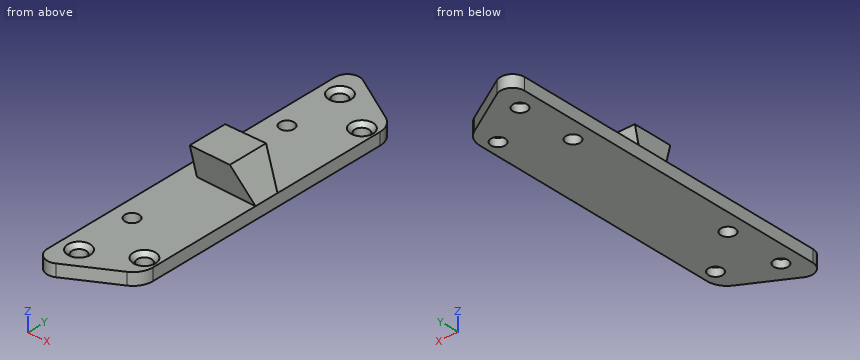
Autodesk Inventor part; units mm, degrees
ref_plane "Plano de trabajo1" through (130.1908, -31.0595, 0) normal (1, 0, 0) x (0, 0, -1)
ref_plane "YZ Plane" through (0, 0, 0) normal (1, 0, 0) x (0, 1, 0)
ref_plane "XZ Plane" through (0, 0, 0) normal (0, 1, 0) x (-1, 0, 0)
sketch "Boceto1" plane through (0, 0, 0) normal (0, 0, 1) x (1, 0, 0)
  line L0 (134.9, 24.045) -> (134.9, 29.745)
  arc A0 (134.9, 24.045) -> (137.5, 24.045) centre (136.2, 24.045) ccw
  line L1 (137.5, 29.745) -> (137.5, 24.045)
  circle A1 centre (136.2, 29.745) radius 1.3 construction
  line L2 (126.9, 35.7) -> (126.9, 21.2)
  line L3 (123.9, 21.2) -> (123.9, 35.7)
  circle A2 centre (125.4, 35.7) radius 1.5 construction
  circle A3 centre (125.4, 21.2) radius 1.5 construction
  line L4 (126.8891, -21.2025) -> (126.8816, -35.7004)
  circle A4 centre (125.3854, -21.2022) radius 1.5037 construction
  line L5 (123.8816, -35.6996) -> (123.8816, -21.2019)
  circle A5 centre (125.3816, -35.6996) radius 1.5 construction
  circle A6 centre (136.1847, -29.7501) radius 1.3 construction
  line L6 (137.4876, -24.0508) -> (137.4847, -29.7508)
  arc A7 (137.4876, -24.0508) -> (134.8876, -24.0494) centre (136.1876, -24.0501) ccw
  line L7 (134.8847, -29.7494) -> (134.8876, -24.0494)
  line L8 (120.8816, 55.9985) -> (120.8816, -0.0015)
  line L9 (139.5, 56.008) -> (139.5, -0.0015)
  line L10 (50.0101, -56.038) -> (139.5, -55.992)
  line L11 (139.5, 56.008) -> (49.9528, 55.962)
  line L12 (136.8302, -30.8785) -> (126.1265, -37.0016) construction
  line L13 (136.9827, -35.3995) -> (125.3713, -42.0418)
  arc A8 (192.3943, -3.7013) -> (191.4002, 0.0347) centre (191.4012, -1.9653) ccw
  line L14 (120.8816, -0.0015) -> (120.8816, -39.4378)
  line L15 (139.5, -0.0015) -> (139.5, -31.0595)
  arc A9 (120.8816, -39.4378) -> (125.3713, -42.0418) centre (123.8816, -39.4378) ccw
  arc A10 (136.9827, -35.3995) -> (139.5, -31.0595) centre (134.5, -31.0595) ccw
  line L16 (139.5, -0.0015) -> (120.8816, -0.0015) construction
  line L17 (136.9827, 35.3964) -> (125.3713, 42.0388)
  arc A11 (125.3713, 42.0388) -> (120.8816, 39.4347) centre (123.8816, 39.4347) ccw
  arc A12 (139.5, 31.0564) -> (136.9827, 35.3964) centre (134.5, 31.0564) ccw
  line L18 (137.2847, -29.7507) -> (137.2876, -24.0507)
  arc A13 (137.2876, -24.0507) -> (135.0876, -24.0495) centre (136.1876, -24.0501) ccw
  line L19 (135.0876, -24.0495) -> (135.0847, -29.7495)
  arc A14 (135.0847, -29.7495) -> (137.2847, -29.7507) centre (136.1847, -29.7501) ccw
  line L20 (126.6816, -35.7003) -> (126.6891, -21.2024)
  arc A15 (126.6891, -21.2024) -> (124.0816, -21.2022) centre (125.3854, -21.2022) ccw
  line L21 (124.0816, -21.2022) -> (124.0816, -35.6996)
  arc A16 (124.0816, -35.6996) -> (126.6816, -35.7003) centre (125.3816, -35.6996) ccw
  arc A17 (135.1, 24.045) -> (137.3, 24.045) centre (136.2, 24.045) ccw
  line L22 (135.1, 24.045) -> (135.1, 29.745)
  arc A18 (137.3, 29.745) -> (135.1, 29.745) centre (136.2, 29.745) ccw
  line L23 (137.3, 29.745) -> (137.3, 24.045)
  line L24 (126.7, 21.2) -> (126.7, 35.7)
  arc A19 (126.7, 35.7) -> (124.1, 35.7) centre (125.4, 35.7) ccw
  line L25 (124.1, 35.7) -> (124.1, 21.2)
  arc A20 (124.1, 21.2) -> (126.7, 21.2) centre (125.4, 21.2) ccw
  circle A21 centre (125.3816, -35.6996) radius 1.75
  circle A22 centre (136.1847, -29.7501) radius 1.75
  circle A23 centre (125.4, 35.7) radius 1.75
  circle A24 centre (136.2, 29.745) radius 1.75
  circle A25 centre (125.4, 21.2) radius 1.75
  circle A26 centre (125.3854, -21.2022) radius 1.75
  point P0 (0, 0)
  point P1 (120.8816, -56.0015)
  point P2 (139.5, -33.9595)
  point P3 (120.8816, -44.6101)
  point P4 (126.7, 34.5285)
  point P5 (124.1, 34.5285)
  point P6 (137.3, 28.3839)
  point P7 (135.1, 28.3839)
  point P8 (124.0816, -34.5281)
  point P9 (126.6823, -34.5287)
  point P10 (135.0854, -28.3885)
  point P11 (137.2854, -28.3896)
  dimension "d0" = 3
  dimension "d1" = 2
  dimension "d2" = 4
  dimension "d3" = 2
  dimension "d4" = 3
  dimension "d5" = 5
  dimension "d8" = 0.2
  dimension "d9" = 0.2
  dimension "d10" = 0.2
  dimension "d11" = 0.2
  dimension "d14" = 3.5
  dimension "d15" = 3.5
  dimension "d16" = 3.5
  dimension "d17" = 3.5
  dimension "d18" = 3.5
  dimension "d19" = 3.5
extrude "Extrusión1" add sketch "Boceto1" along normal blind 3 contours L0 A24 L22 A17 L23 L1 A0 | A24 L23 A18 L22 | A24 L23 A17 L22 | L22 A18 L23 A24 | L2 A25 L24 A23 | A23 L24 A19 L25 | A23 L25 A19 L24 | L24 A25 L25 A23 | L25 A25 L3 A23 | L4 A21 L20 A26 | A21 L21 A16 L20 | L20 A21 L21 A26 | L20 A16 L21 A21 | L21 A21 L5 A26 | L6 A22 L18 A13 L19 L7 A7 | A22 L19 A14 L18 | A22 L19 A13 L18 | L18 A14 L19 A22 | A11 L17 A12 L9 L15 A10 L13 A9 L14 L8
extrude "Extrusión2" [suppressed]
sketch "Boceto2" plane through (0, 0, 3) normal (0, 0, 1) x (1, 0, 0)
  point P0 (0, 0)
  point P1 (125.4, 35.7)
  point P2 (136.2, 29.745)
  point P3 (125.4, 21.2)
  point P4 (136.1847, -29.7501)
  point P5 (125.3854, -21.2022)
  point P6 (125.3816, -35.6996)
hole "Agujero1" at (125.4, 35.7, 3) at (136.2, 29.745, 3) at (136.1847, -29.7501, 3) at (125.3816, -35.6996, 3) direction (0, 0, -1) diameter 3.5 end through all countersink diameter 5.5 countersink angle 90
ref_plane "Plano de trabajo1" through (130.1908, -31.0595, 0) normal (1, 0, 0) x (0, 0, -1)
sketch "Boceto3" plane through (139.5, -31.0595, 0) normal (1, 0, 0) x (0, 0, -1)
  line L0 (-3, 31.0579) -> (-11, 31.0579) construction
  line L1 (-11, 26.0579) -> (-11, 36.0579)
  line L2 (-11, 26.0579) -> (-3, 28.0579)
  line L3 (-11, 36.0579) -> (-3, 34.0579)
  line L4 (0, 0) -> (0, 62.1159)
  line L5 (-3, 28.0579) -> (0, 28.0579)
  line L6 (-3, 34.0579) -> (0, 34.0579)
  line L7 (-3, 0) -> (-3, 28.0579)
  line L8 (-3, 34.0579) -> (-3, 62.1159)
  line L9 (-3, 0) -> (-3, 28.0579)
  line L10 (-3, 34.0579) -> (-3, 62.1159)
  point P0 (0, 31.0595)
  dimension "d27" = 8
  dimension "d28" = 10
  dimension "d29" = 6
extrude "Extrusión3" add sketch "Boceto3" against normal blind 14.618 draft -0.5
sketch "Boceto4" plane through (0, 0, 0) normal (0, 1, 0) x (-1, 0, 0)
  line L0 (-124.882, 10.8724) -> (-124.882, 3.0157)
  line L1 (-139.5, 3) -> (-124.882, 3.0157)
  line L2 (-139.5, 11) -> (-139.5, 3)
  line L3 (-139.5, 11) -> (-124.882, 10.8724)
  line L4 (-139.5, 3) -> (-134.9044, 10.9599)
  point P0 (0, 0)
  dimension "d32" = 30
extrude "Extrusión4" cut sketch "Boceto4" along normal through all both and the other way through all contours L4 L2 L3
properties part number "AcopleCamara-part1"
Verification items for the finished model (mm, model axes). Coordinates: 2 decimals unless noted, no trailing zeros. Order: outer loops, then holes, each group sorted by start corner. A loop starts at its lowest first (then second) coordinate and runs counter-clockwise, first axis right, second up. Notation, with made-up numbers: (4, 5) -> (29, 5) arc R18 ccw to (29, 9) -> close; hole circle Ø7 at (-3.5, 1.5). An arc over 180 degrees is marked (long way). Put each result on its own line as item: value. Start each with the question number.
1. Material ranges on L1, parallel to Y at x = 125.4, z = 0.8; L2, parallel to Y at x = 126, z = 2.75; L3, parallel to Z at x = 134, y = 1.5, recorded low to high. Write a range as [from, to].
2. Cross-section at B-B, the plane y = 1. Record the boundary of the cut face in (x, z).
3. Go/stop test with flat-tipped pins: pin 1 Ø4 at (x, y) = (125.4, 21.2) entering from +Z; pin 2 Ø1.5 at (x, y) = (127, 0) entering from -Z; pin 3 Ø4 at (y, z) = (2.5, 7) entering from -X; pin 4 Ø3 at (x, y) = (125.4, 35.7) entering from +Z. Record where each tip stops, or that it passes through.
4. Cross-section at A-A, the plane y = 21.2. Record the boundary of the cut face in (x, z).
5. Cross-section at D-D, the plane z = 5. Record the boundary of the cut face in (x, y), then the cut area to 3 significant figures.
Computed:
1. L1: [-42.03, -37.45], [-33.95, -22.95], [-19.45, 19.45], [22.95, 33.95], [37.45, 42.02]
1. L2: [-41.68, -38.12], [-33.28, -22.84], [-19.56, 19.56], [22.84, 33.27], [38.13, 41.68]
1. L3: [0, 10.95]
2. outline: (120.88, 0) -> (139.5, 0) -> (139.5, 3) -> (134.9, 10.96) -> (124.88, 10.87) -> (124.88, 3) -> (120.88, 3) -> close
3. pin 1: z = 3
3. pin 2: z = 0
3. pin 3: x = 124.88
3. pin 4: through
4. outline: (120.88, 0) -> (123.65, 0) -> (123.65, 3) -> (120.88, 3) -> close; (127.15, 0) -> (139.5, 0) -> (139.5, 3) -> (127.15, 3) -> close
5. outline: (124.88, -3.37) -> (138.35, -3.49) -> (138.35, 3.49) -> (124.88, 3.37) -> close
5. area: 92.3 mm2
